Geometry: see drawing. Coordinates: mm, zero at the bounding-box minimum. A direction names the side the tool comes from. Give positions to 0.01 mm unless a question says otherwise; leave off trailing zeros. Write each loop counter-clockwise with the first axis right and the second up, starting at its lowest first coordinate (ties: lowest second). Pieces come first, ordered by that corner, then holes. Notation, with made-up numbers: M 53.5,-35 L 90.5,-35 A15 ccw 90.5,-15 Z; hole C 62.5,41 d8. An arc over 180 degrees is marked long. Use one line per item in the form item = value. Start each with the question number.
Item 1: Section query D-D on z = 67. Return loops of the section in (x, y).
Item 2: Section query C-C on x = 23. Return loops of the section in (y, z), then the cut area to 3 significant figures.
Item 3: Material intervals for line 1 along Y through (x, z) = (12, 33.5); line 2 along Y through (x, z) = (12.5, 5); line 3 along X through (y, z) = (17.5, 22.75), sorted ascending. Write a range as from..to.
Item 4: Access query for the marked faces 1, 2 and 3. Directions: +Z, -Z, +X, -X, +Y, -Y. A direction counts if a zero-diameter tool reaches every point of the face in a straight line with its end or side. Return the directions, or none.
Item 5: Section query A-A on z = 5. Return loops of the section in (x, y).
Item 6: Section query B-B on y = 4. Return loops of the section in (x, z), then the cut area to 3 significant figures.
Item 7: Contact query for flat-ended pins moving along their axis: P1, Ø1.6, axis at x = 15, y = 0.5, coming from the +Z side; P2, Ø7.5, axis at x = 13.5, z = 39.5, coming from the -Y side; P3, Ø3, axis at y = 4, z = 15, coming from the +X side; P4, Ø10, axis at x = 17, y = 16.5, coming from the +Z side. Output: stop coordinate, or through.
Item 8: Pull-direction query (Y, two-part tool) for the marked faces 4, 5 and 6; classes: released by +Y, released by -Y, zero draft, split by the parting line, or undercut.
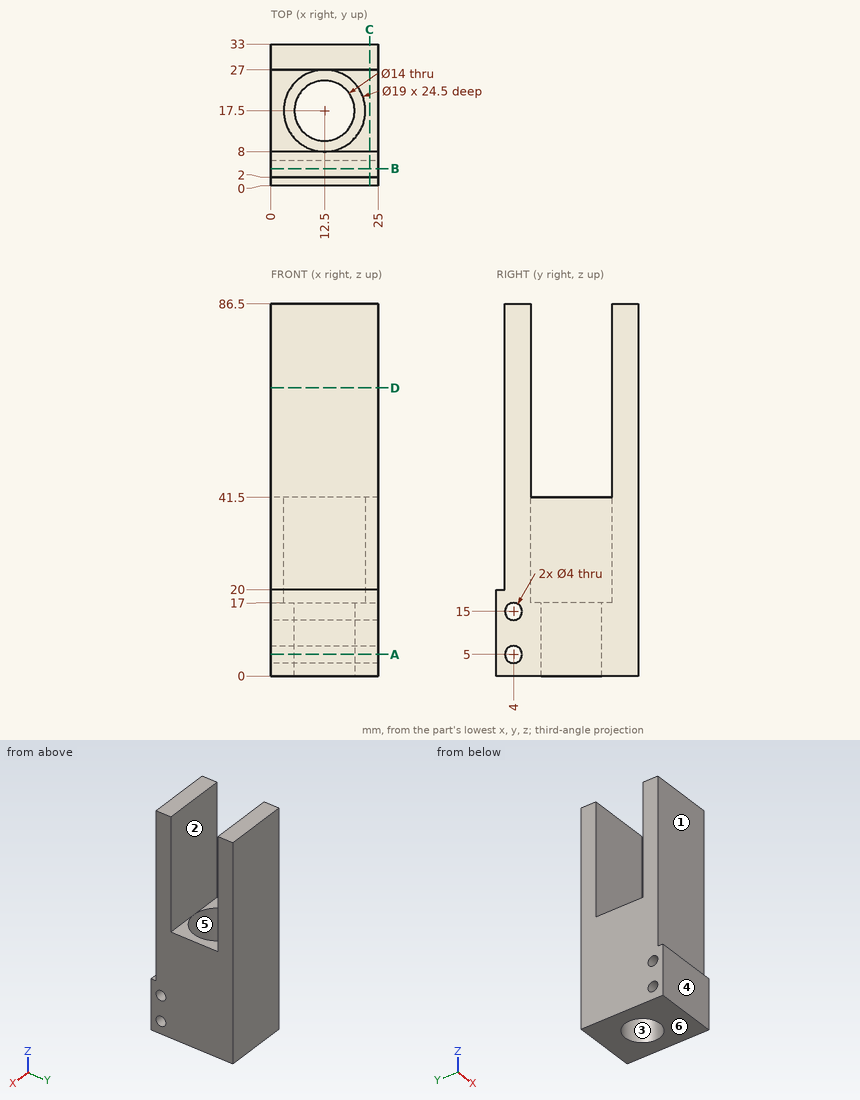
Answer sheet:
q1.outline = M 0,2 L 25,2 L 25,8 L 0,8 Z; M 0,27 L 25,27 L 25,33 L 0,33 Z
q2.outline = M 0,0 L 33,0 L 33,86.5 L 27,86.5 L 27,41.5 L 8,41.5 L 8,86.5 L 2,86.5 L 2,20 L 0,20 Z; hole C 4,5 d4; hole C 4,15 d4
q2.area = 1,840 mm2
q3.line_1 = 2..8.01, 26.99..33
q3.line_2 = 0..2, 6..10.5, 24.5..33
q3.line_3 = 0..3, 22..25
q4.face_1 = +Z, +X, -X, -Y
q4.face_2 = +Z, +X, -X
q4.face_3 = +Z, -Z
q5.outline = M 0,0 L 25,0 L 25,2 L 0,2 Z; M 0,6 L 25,6 L 25,33 L 0,33 Z; hole C 12.5,17.5 d14
q6.outline = M 0,0 L 25,0 L 25,3 L 0,3 Z; M 0,7 L 25,7 L 25,13 L 0,13 Z; M 0,17 L 25,17 L 25,86.5 L 0,86.5 Z
q6.area = 1,960 mm2
q7.P1 = 20
q7.P2 = 2
q7.P3 = through
q7.P4 = 41.5
q8.face_4 = released by -Y
q8.face_5 = undercut
q8.face_6 = zero draft
